```python
from build123d import *

# Parameters (mm, degrees)
F0_W     = 781.05
F0_H     = 400.05
F0_R     = 6.35
F1_DEPTH = 3.175


with BuildPart() as f1:
    # F0 (on Top) → F1 (new body)
    with BuildSketch(Plane.XY):
        with Locations((390.525, 200.025)):
            Rectangle(F0_W, F0_H)
        with Locations((28.575, 25.4)):
            Circle(F0_R, mode=Mode.SUBTRACT)
        with Locations((149.225, 25.4)):
            Circle(F0_R, mode=Mode.SUBTRACT)
        with Locations((269.875, 25.4)):
            Circle(F0_R, mode=Mode.SUBTRACT)
        with Locations((28.575, 139.7)):
            Circle(F0_R, mode=Mode.SUBTRACT)
        with Locations((390.525, 25.4)):
            Circle(F0_R, mode=Mode.SUBTRACT)
        with Locations((511.175, 25.4)):
            Circle(F0_R, mode=Mode.SUBTRACT)
        with Locations((631.825, 25.4)):
            Circle(F0_R, mode=Mode.SUBTRACT)
        with Locations((752.475, 25.4)):
            Circle(F0_R, mode=Mode.SUBTRACT)
        with BuildLine():
            Line((631.825, 50.412805), (149.225, 50.412805))
            ThreePointArc((149.225, 50.412805), (113.303976, 65.29178), (98.425, 101.212805))
            Line((98.425, 101.212805), (98.425, 298.062805))
            ThreePointArc((98.425, 298.062805), (113.303976, 333.983829), (149.225, 348.862805))
            Line((149.225, 348.862805), (631.825, 348.862805))
            ThreePointArc((631.825, 348.862805), (667.746024, 333.983829), (682.625, 298.062805))
            Line((682.625, 298.062805), (682.625, 101.212805))
            ThreePointArc((682.625, 101.212805), (667.746024, 65.29178), (631.825, 50.412805))
        make_face(mode=Mode.SUBTRACT)
        with Locations((752.475, 139.7)):
            Circle(F0_R, mode=Mode.SUBTRACT)
        with Locations((28.575, 260.35)):
            Circle(F0_R, mode=Mode.SUBTRACT)
        with Locations((28.575, 374.65)):
            Circle(F0_R, mode=Mode.SUBTRACT)
        with Locations((149.225, 374.65)):
            Circle(F0_R, mode=Mode.SUBTRACT)
        with Locations((269.875, 374.65)):
            Circle(F0_R, mode=Mode.SUBTRACT)
        with Locations((752.475, 260.35)):
            Circle(F0_R, mode=Mode.SUBTRACT)
        with Locations((390.525, 374.65)):
            Circle(F0_R, mode=Mode.SUBTRACT)
        with Locations((511.175, 374.65)):
            Circle(F0_R, mode=Mode.SUBTRACT)
        with Locations((631.825, 374.65)):
            Circle(F0_R, mode=Mode.SUBTRACT)
        with Locations((752.475, 374.65)):
            Circle(F0_R, mode=Mode.SUBTRACT)
    extrude(amount=F1_DEPTH)


solid = f1.part
```
Geometry check sheet. Reference: the model listing, model coordinates, mm. A direction names the side the tool comes from. Give positions to 0.01 mm unless a question says otherwise; leave off trailing zeros. Write each loop counter-clockwise with the first axis right and the second up, starting at its lowest first coordinate (ties: lowest second). Pieces come first, ordered by that corner, then holes.
1) Release check for a two-part mould opening along Y. For faces 1 (the flat face through (385, 381, 3.175)), 2 (the cylindrical face through (112.911, 333.587, 1.565)) record: pulls with the +Y half, pulls with the -Y half, needs draft (parallel to the pull), parting line crosses it, or undercut.
2) Material ranges on L1, parallel to X at y = 260.35, z = 1.05 (3 decimals); L2, parallel to Y at x = 450.5, z = 0.8; L3, parallel to X at y = 233, z = 1.3 (3 decimals), recorded low to high.
3) Access from +Z, -Z, +X, -X, +Y, -Y to the whole of each face (thin tool, end or side, straight path). Record for faces 3 (the cylindrical face through (113.7, 64.9, 1.6)), 4 (the flat face through (385, 381, 0)).
4) Gauge pin test, flat end, axial feed: pin 1 (10 mm diameter, centred on x = 752.475, y = 374.65, fed in from -Z). Record the tip position at first contact, or that the pin passes through.
5) Section check C-C, the plane z = 0.8. State how many separate pieces and enclosed holes the cut face has, and give its area (3 significant figures).
6) Section check A-A, the plane x = 181.5. Record the boundary of the cut face in (y, z) (3 decimals), and give its area (3 significant figures).
7) Section check B-B, the plane y = 240. Record the boundary of the cut face in (x, z) (3 decimals).
Computed:
1. face 1: needs draft
1. face 2: undercut
2. L1: x = 0 to 22.225, 34.925 to 98.425, 682.625 to 746.125, 758.825 to 781.05
2. L2: y = 0 to 50.41, 348.86 to 400.05
2. L3: x = 0 to 98.425, 682.625 to 781.05
3. face 3: +Z, -Z
3. face 4: -Z, +X, -X, +Y, -Y
4. pin 1: passes through
5. separate pieces: 1
5. enclosed holes: 19
5. area: 138,000 mm2
6. outline: (0, 0) - (50.413, 0) - (50.413, 3.175) - (0, 3.175) - close; (348.863, 0) - (400.05, 0) - (400.05, 3.175) - (348.863, 3.175) - close
6. area: 323 mm2
7. outline: (0, 0) - (98.425, 0) - (98.425, 3.175) - (0, 3.175) - close; (682.625, 0) - (781.05, 0) - (781.05, 3.175) - (682.625, 3.175) - close
